```python
from build123d import *

# Parameters (mm, degrees)
BOSS_EXTRUDE1_DEPTH               = 12.7
F_1_4_20_TAPPED_HOLE1_D           = 5.1054
F_1_4_20_TAPPED_HOLE1_CSINK_D     = 7.62
F_1_4_20_TAPPED_HOLE1_CSINK_ANGLE = 100
F_1_4_0_25_DIAMETER_HOLE1_D       = 6.35
F_1_4_0_25_DIAMETER_HOLE1_DEPTH   = 19.05
F_1_4_0_25_DIAMETER_HOLE1_TIP     = 1.907732465


with BuildPart() as part:
    # Sketch1 → Boss-Extrude1 (new body)
    with BuildSketch(Plane.XY):
        Polygon((-20, 0), (20, 0), (20, 20), (10, 20), (10, 200), (-10, 200), (-10, 20), (-20, 20), align=None)
    extrude(amount=BOSS_EXTRUDE1_DEPTH)

    # 1/4-20 Tapped Hole1 (through all)
    with Locations(Plane(origin=(0, 0, 0), x_dir=(-1, 0, 0), z_dir=(0, 0, -1))):
        with Locations((0, 168.25), (0, 130.15)):
            CounterSinkHole(F_1_4_20_TAPPED_HOLE1_D / 2, F_1_4_20_TAPPED_HOLE1_CSINK_D / 2, counter_sink_angle=F_1_4_20_TAPPED_HOLE1_CSINK_ANGLE)

    # 1/4 (0.25) Diameter Hole1
    with Locations(Plane(origin=(0, 0, 0), x_dir=(-1, 0, 0), z_dir=(0, 0, -1))):
        with Locations((14.5, 9), (-14.5, 9)):
            Hole(F_1_4_0_25_DIAMETER_HOLE1_D / 2, depth=F_1_4_0_25_DIAMETER_HOLE1_DEPTH)
            with Locations((0, 0, -(F_1_4_0_25_DIAMETER_HOLE1_DEPTH + F_1_4_0_25_DIAMETER_HOLE1_TIP / 2))):  # 118° drill point
                Cone(0, F_1_4_0_25_DIAMETER_HOLE1_D / 2, F_1_4_0_25_DIAMETER_HOLE1_TIP, mode=Mode.SUBTRACT)


solid = part.part
```
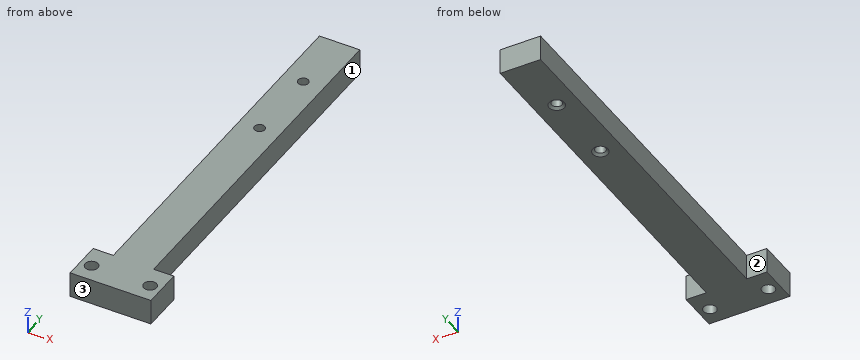
Verification items for the finished model (mm, model axes). Face numbers are marked on the shaded views. A direction names the side the tool comes from. Give positions to 0.01 mm unless a question says otherwise; leave off trailing zeros. Order: outer loops, then holes, each group sorted by start corner. A loop starts at its lowest first (then second) coordinate and runs counter-clockwise, first axis right, second up. Notation, with made-up numbers: (40.25, -3.5) - (50.25, -3.5) arc R30 ccw to (50.25, 26.5) - close; hole circle Ø4 at (58, -24.5). An arc over 180 degrees is marked (long way). Answer as CSV lines item,"result". Start each with the question number.
Item 1: Gauge pin test, flat ends, axial feed: pin 1 (3 mm diameter, centred on y = 82.5, z = 7.5, fed in from -X); pin 2 (5 mm diameter, centred on x = -13.5, z = 7.5, fed in from +Y); pin 3 (1.5 mm diameter, centred on y = 74.5, z = 2.5, fed in from +X). Record the tip position at first contact, or that the pin passes through.
Item 2: Section check B-B, the plane y = 9. Record the boundary of the cut face in (x, z) (3 decimals).
Item 3: Section check D-D, the plane x = 0. Record the boundary of the cut face in (y, z) (3 decimals), plus the area to 3 significant figures.
Item 4: Access from +Z, -Z, +X, -X, +Y, -Y to the whole of each face (thin tool, end or side, straight path). Record for the marked faces 1, 2 and 3.
Item 5: Section check C-C, the plane z = 8. Record the boundary of the cut face in (x, y) (3 decimals).
Item 6: Material ranges on L1, parallel to Y at x = 14.5, z = 8 (3 decimals); L2, parallel to Y at x = 0, z = 4.5; L3, parallel to X at y = 130.15, z = 7.5, recorded low to high.
Item 7: Section check A-A, the plane y = 168.25. Record the boundary of the cut face in (x, z) (3 decimals).
Filled in:
1,pin 1,"x = -10"
1,pin 2,"y = 20"
1,pin 3,"x = 10"
2,outline,"(-20, 0) - (-17.675, 0) - (-17.675, 12.7) - (-20, 12.7) - close; (-11.325, 0) - (11.325, 0) - (11.325, 12.7) - (-11.325, 12.7) - close; (17.675, 0) - (20, 0) - (20, 12.7) - (17.675, 12.7) - close"
3,outline,"(0, 0) - (126.34, 0) - (127.597, 1.055) - (127.597, 12.7) - (0, 12.7) - close; (132.703, 1.055) - (133.96, 0) - (164.44, 0) - (165.697, 1.055) - (165.697, 12.7) - (132.703, 12.7) - close; (170.803, 1.055) - (172.06, 0) - (200, 0) - (200, 12.7) - (170.803, 12.7) - close"
3,area,"2,410 mm^2"
4,face 1,"+Z, -Z, +X, +Y"
4,face 2,"+Z, -Z, -X, +Y"
4,face 3,"+Z, -Z, +X, -X, -Y"
5,outline,"(-20, 0) - (20, 0) - (20, 20) - (10, 20) - (10, 200) - (-10, 200) - (-10, 20) - (-20, 20) - close; hole circle Ø6.35 at (-14.5, 9); hole circle Ø5.105 at (0, 130.15); hole circle Ø5.105 at (0, 168.25); hole circle Ø6.35 at (14.5, 9)"
6,L1,"0 to 5.825, 12.175 to 20"
6,L2,"0 to 127.6, 132.7 to 165.7, 170.8 to 200"
6,L3,"-10 to -2.55, 2.55 to 10"
7,outline,"(-10, 0) - (-3.81, 0) - (-2.553, 1.055) - (-2.553, 12.7) - (-10, 12.7) - close; (2.553, 1.055) - (3.81, 0) - (10, 0) - (10, 12.7) - (2.553, 12.7) - close"
